from build123d import *

# Parameters (mm, degrees)
BOSS_EXTRUDE1_DEPTH = 6.35
SKETCH2_R           = 1.651
CUT_EXTRUDE1_DEPTH  = 6.35


with BuildPart() as part:
    # Sketch1 → Boss-Extrude1 (new body)
    with BuildSketch(Plane(origin=(0, 0, 0), x_dir=(1, 0, 0), z_dir=(0, 1, 0))):
        with BuildLine():
            Line((-15.08125, 0), (-34.13125, 0))
            Line((-34.13125, 0), (-34.13125, 3.175))
            Line((-34.13125, 3.175), (-18.25625, 3.175))
            ThreePointArc((-18.25625, 3.175), (0, 18.530280329), (18.25625, 3.175))
            Line((18.25625, 3.175), (34.13125, 3.175))
            Line((34.13125, 3.175), (34.13125, 0))
            Line((34.13125, 0), (15.08125, 0))
            ThreePointArc((15.08125, 0), (0, 15.08125), (-15.08125, 0))
        make_face()
    extrude(amount=BOSS_EXTRUDE1_DEPTH)

    # Sketch2 → Cut-Extrude1 (cut)
    with BuildSketch(Plane(origin=(0, 0, -3.175), x_dir=(-1, 0, 0), z_dir=(0, 0, -1))):
        with Locations((26.19375, 3.175)):
            Circle(SKETCH2_R)
    cut_extrude1 = extrude(amount=-CUT_EXTRUDE1_DEPTH, mode=Mode.SUBTRACT)

    # Mirror1: Cut-Extrude1 across plane
    add(cut_extrude1.mirror(Plane(origin=(0, 0, 0), x_dir=(0, 0, 1), z_dir=(1, 0, 0))), mode=Mode.SUBTRACT)


solid = part.part
The listing builds one solid part. Answer for the finished solid, in the listing's coordinates (mm). A direction names the side the tool comes from. Give positions to 0.01 mm unless a question says otherwise; leave off trailing zeros. Order: outer loops, then holes, each group sorted by start corner. A loop starts at its lowest first (then second) coordinate and runs counter-clockwise, first axis right, second up. Notation, with made-up numbers: (-11.75, 57) - (34.25, 57) arc R12 ccw to (34.25, 72) - close; hole circle Ø2 at (4.5, -28.75). An arc over 180 degrees is marked (long way). Use one line per item in the form item = value.
1) Find section A-A on z = -2. Determine the outline of the cut face in (x, y) (3 decimals).
Verdict:
outline = (-34.131, 0) - (-14.948, 0) - (-14.948, 6.35) - (-34.131, 6.35) - close; (14.948, 0) - (34.131, 0) - (34.131, 6.35) - (14.948, 6.35) - close; hole circle Ø3.302 at (-26.194, 3.175); hole circle Ø3.302 at (26.194, 3.175)
2) The mould has two halves that part along X. Classify faces 3 (the cylindrical face through (-27.77, 3.67, -1.61)), 4 (the flat face through (-34.131, 3, -2)), 5 (the flat face through (-28, 3, -3.175)): released by +X, released by -X, zero draft, split by the parting line, or undercut.
Verdict:
face_3 = undercut
face_4 = released by -X
face_5 = zero draft
3) Find section C-C on z = -9.75. Determine the outline of the cut face in (x, y).
Verdict:
outline = (-15.76, 0) - (-11.51, 0) - (-11.51, 6.35) - (-15.76, 6.35) - close; (11.51, 0) - (15.76, 0) - (15.76, 6.35) - (11.51, 6.35) - close
4) Find section B-B on y = 2.25. Determine the outline of the cut face in (x, z) (1 decimal), and give its area (3 significant figures).
Verdict:
outline = (-34.1, -3.2) - (-27.6, -3.2) - (-27.6, 0) - (-34.1, 0) - close; (-24.8, -3.2) - (-18.3, -3.2) arc R18.5 ccw to (18.3, -3.2) - (24.8, -3.2) - (24.8, 0) - (15.1, 0) arc R15.1 cw to (-15.1, 0) - (-24.8, 0) - close; (27.6, -3.2) - (34.1, -3.2) - (34.1, 0) - (27.6, 0) - close
area = 264 mm^2
5) Each of these flat-tipped pins is pushed along its axis until it touches: pin 1 (3 mm diameter, centred on x = 24, y = 3.5, fed in from -Z) (3 decimals); pin 2 (2 mm diameter, centred on y = 4, z = -9.5, fed in from +X); pin 3 (1.5 mm diameter, centred on y = 4.5, z = -14, fed in from +X). Where does it stop, or does it pass through?
Verdict:
pin_1 = -3.175
pin_2 = 16.47
pin_3 = 12.95
6) For faces 1 (the flat face through (28, 3, -3.175)), 2 (the cylindrical face through (-0.363, 3.131, -18.527)), determine the directions among +Z, -Z, +X, -X, +Y, -Y from which every point of the face is accessible in a straight line to the end or side of a thin tool.
Verdict:
face_1 = -Z, +X, +Y, -Y
face_2 = -Z, +Y, -Y
7) Consider probe 1 along Z at (x, y) = (-20, 1) (3 decimals); probe 2 along X at (y, z) = (4.5, -5); probe 3 along X at (y, z) = (3.75, -1). Determine where each line is inside the solid, lowest interval first. Write a range as [from, to].
Verdict:
probe_1 = [-3.175, 0]
probe_2 = [-17.84, -14.23], [14.23, 17.84]
probe_3 = [-34.13, -27.74], [-24.65, -15.05], [15.05, 24.65], [27.74, 34.13]
8) Find section D-D on x = 0. Determine the outline of the cut face in (y, z).
Verdict:
outline = (0, -18.53) - (6.35, -18.53) - (6.35, -15.08) - (0, -15.08) - close
